```python
from build123d import *

# Parameters (mm, degrees)
SKETCH2_W               = 50
SKETCH2_H               = 45
SKETCH2_W_2             = 45
SKETCH2_H_2             = 40
BOSS_EXTRUDE1_DEPTH     = 30
SKETCH4_R               = 9.5
CUT_EXTRUDE1_DEPTH      = 1
CUT_EXTRUDE1_DEPTH_BACK = 46
SKETCH5_R               = 9.5
CUT_EXTRUDE2_DEPTH      = 1
CUT_EXTRUDE2_DEPTH_BACK = 51


with BuildPart() as part:
    # Sketch2 → Boss-Extrude1 (new body)
    with BuildSketch(Plane(origin=(0, 0, 0), x_dir=(1, 0, 0), z_dir=(0, 1, 0))):
        Rectangle(SKETCH2_W, SKETCH2_H)
        Rectangle(SKETCH2_W_2, SKETCH2_H_2, mode=Mode.SUBTRACT)
    extrude(amount=BOSS_EXTRUDE1_DEPTH)

    # Sketch4 → Cut-Extrude1 (cut, two sides)
    with BuildSketch(Plane.XY.offset(22.5)) as cut_extrude1_sk:
        with Locations((0, 15)):
            Circle(SKETCH4_R)
    extrude(amount=CUT_EXTRUDE1_DEPTH, mode=Mode.SUBTRACT)
    extrude(cut_extrude1_sk.sketch, amount=-CUT_EXTRUDE1_DEPTH_BACK, mode=Mode.SUBTRACT)

    # Sketch5 → Cut-Extrude2 (cut, two sides)
    with BuildSketch(Plane.ZY.offset(25)) as cut_extrude2_sk:
        with Locations((0, 15)):
            Circle(SKETCH5_R)
    extrude(amount=CUT_EXTRUDE2_DEPTH, mode=Mode.SUBTRACT)
    extrude(cut_extrude2_sk.sketch, amount=-CUT_EXTRUDE2_DEPTH_BACK, mode=Mode.SUBTRACT)


solid = part.part
```
Geometry: final body of the model. Coordinates: model frame, mm. A direction names the side the tool comes from. Round coordinates to 2 decimals unless told otherwise and drop trailing zeros. Write each loop counter-clockwise with the first axis right and the second up, starting at its lowest first coordinate (ties: lowest second). Pieces come first, ordered by that corner, then holes. Notation, with made-up numbers: (7, 89.5) -> (62, 89.5) arc R32 ccw to (62, 123.5) -> close; hole circle Ø4 at (77, 74.5). An arc over 180 degrees is marked (long way). Return JSON: item names as keys, results as strings.
Q1. First-contact query: pin 1 Ø15 at (y, z) = (22, -2.5) entering from +X. Flat tip, straight axial feed; report the tip coordinate or a pass-through.
From the geometry:
{"pin 1": "x = 25"}
Q2. Section D-D on z = 11.5. Return the cut outline in (x, y), and give its area (3 significant figures).
From the geometry:
{"outline": "(-25, 0) -> (-22.5, 0) -> (-22.5, 30) -> (-25, 30) -> close; (22.5, 0) -> (25, 0) -> (25, 30) -> (22.5, 30) -> close", "area": "150 mm2"}
Q3. Section C-C on x = -20. Return the cut outline in (y, z).
From the geometry:
{"outline": "(0, -22.5) -> (30, -22.5) -> (30, -20) -> (0, -20) -> close; (0, 20) -> (30, 20) -> (30, 22.5) -> (0, 22.5) -> close"}
Q4. Section A-A on z = 0. Return the cut outline in (x, y), and give its area (3 significant figures).
From the geometry:
{"outline": "(-25, 0) -> (-22.5, 0) -> (-22.5, 5.5) -> (-25, 5.5) -> close; (-25, 24.5) -> (-22.5, 24.5) -> (-22.5, 30) -> (-25, 30) -> close; (22.5, 0) -> (25, 0) -> (25, 5.5) -> (22.5, 5.5) -> close; (22.5, 24.5) -> (25, 24.5) -> (25, 30) -> (22.5, 30) -> close", "area": "55.0 mm2"}
Q5. Ray query, line 1 (X direction, y = 22.75, z = 6); line 2 (Z direction, x = -13.5, y = 10.5); line 3 (Y direction, x = -23, z = 0). Return the intervals inside material, ascending.
From the geometry:
{"line 1": "-25 to -22.5, 22.5 to 25", "line 2": "-22.5 to -20, 20 to 22.5", "line 3": "0 to 5.5, 24.5 to 30"}
Q6. Section B-B on y = 15. Return the cut outline in (x, z).
From the geometry:
{"outline": "(-25, -22.5) -> (-9.5, -22.5) -> (-9.5, -20) -> (-22.5, -20) -> (-22.5, -9.5) -> (-25, -9.5) -> close; (-25, 9.5) -> (-22.5, 9.5) -> (-22.5, 20) -> (-9.5, 20) -> (-9.5, 22.5) -> (-25, 22.5) -> close; (9.5, -22.5) -> (25, -22.5) -> (25, -9.5) -> (22.5, -9.5) -> (22.5, -20) -> (9.5, -20) -> close; (9.5, 20) -> (22.5, 20) -> (22.5, 9.5) -> (25, 9.5) -> (25, 22.5) -> (9.5, 22.5) -> close"}
Q7. Set-up query: faces 5 (the flat face through (22.5, 18.1, 9.2)), 6 (the flat face through (0, 5, 22.5)). Return all of +Z, -Z, +X, -X, +Y, -Y with unobstructed straight access to the full face (end or side cutting, diameter ignored); none if empty.
From the geometry:
{"face 5": "+Y, -Y", "face 6": "+Z, +X, -X, +Y, -Y"}
Q8. Mould query, pull axis Z, two halves, no side actions, for faces 1 (the flat face through (0, 5, -22.5)), 2 (the flat face through (0, 5, 20)), 3 (the flat face through (0, 5, -20)), 4 (the cylindrical face through (9.061, 17.854, 21.268)). Classes: +Z half, -Z half, draft (parallel to the pull), parting line (faces both ways), or undercut.
From the geometry:
{"face 1": "-Z half", "face 2": "undercut", "face 3": "undercut", "face 4": "draft"}
